Autodesk Inventor part; units mm, degrees
ref_plane "b1_XY" through (-12.7, 0, -12.7) normal (1, 0, 0) x (0, 0, -1)
ref_plane "b1_YZ" through (-12.7, 0, -12.7) normal (0, 0, -1) x (0, 1, 0)
ref_plane "b1_ZX" through (-12.7, 0, -12.7) normal (0, 1, 0) x (1, 0, 0)
sketch "Sketch_1" plane through (0, 0, 0) normal (0, 0, 1) x (1, 0, 0)
  arc A0 (-12.6998, -10.5664) -> (-10.5664, -12.6998) centre (-10.5918, -10.5918) ccw
  arc A1 (-9.5504, -12.7) -> (-10.5664, -12.6998) centre (-10.0584, -12.7) ccw
  line L0 (-9.5504, -12.7) -> (-6.3331, -12.7)
  arc A2 (-5.3171, -12.7) -> (-6.3331, -12.7) centre (-5.8251, -12.7) ccw
  line L1 (-5.3171, -12.7) -> (-4.3434, -12.7)
  arc A3 (-4.3434, -12.7) -> (-4.3434, -10.4902) centre (-4.3434, -11.5951) ccw
  line L2 (-4.3434, -10.4902) -> (-6.4748, -10.4902)
  arc A4 (-7.1932, -8.7558) -> (-6.4748, -10.4902) centre (-6.4748, -9.4742) ccw
  line L3 (-7.1932, -8.7558) -> (-3.8632, -5.4257)
  arc A5 (-1.6181, -4.4958) -> (-3.8632, -5.4257) centre (-1.6181, -7.6708) ccw
  line L4 (-1.6181, -4.4958) -> (1.6181, -4.4958)
  arc A6 (3.8632, -5.4257) -> (1.6181, -4.4958) centre (1.6181, -7.6708) ccw
  line L5 (3.8632, -5.4257) -> (7.1932, -8.7558)
  arc A7 (6.4748, -10.4902) -> (7.1932, -8.7558) centre (6.4748, -9.4742) ccw
  line L6 (6.4748, -10.4902) -> (4.3434, -10.4902)
  arc A8 (4.3434, -10.4902) -> (4.3434, -12.7) centre (4.3434, -11.5951) ccw
  line L7 (4.3434, -12.7) -> (5.3171, -12.7)
  arc A9 (6.3331, -12.7) -> (5.3171, -12.7) centre (5.8251, -12.7) ccw
  line L8 (6.3331, -12.7) -> (9.5504, -12.7)
  arc A10 (10.5664, -12.6998) -> (9.5504, -12.7) centre (10.0584, -12.7) ccw
  arc A11 (10.5664, -12.6998) -> (12.6998, -10.5664) centre (10.5918, -10.5918) ccw
  arc A12 (12.7, -9.5504) -> (12.6998, -10.5664) centre (12.7, -10.0584) ccw
  line L9 (12.7, -9.5504) -> (12.7, -6.3331)
  arc A13 (12.7, -5.3171) -> (12.7, -6.3331) centre (12.7, -5.8251) ccw
  line L10 (12.7, -5.3171) -> (12.7, -4.3434)
  arc A14 (12.7, -4.3434) -> (10.4902, -4.3434) centre (11.5951, -4.3434) ccw
  line L11 (10.4902, -4.3434) -> (10.4902, -6.4748)
  arc A15 (8.7558, -7.1932) -> (10.4902, -6.4748) centre (9.4742, -6.4748) ccw
  line L12 (8.7558, -7.1932) -> (5.4257, -3.8632)
  arc A16 (4.4958, -1.6181) -> (5.4257, -3.8632) centre (7.6708, -1.6181) ccw
  line L13 (4.4958, -1.6181) -> (4.4958, 1.6181)
  arc A17 (5.4257, 3.8632) -> (4.4958, 1.6181) centre (7.6708, 1.6181) ccw
  line L14 (5.4257, 3.8632) -> (8.7558, 7.1932)
  arc A18 (10.4902, 6.4748) -> (8.7558, 7.1932) centre (9.4742, 6.4748) ccw
  line L15 (10.4902, 6.4748) -> (10.4902, 4.3434)
  arc A19 (10.4902, 4.3434) -> (12.7, 4.3434) centre (11.5951, 4.3434) ccw
  line L16 (12.7, 4.3434) -> (12.7, 5.3171)
  arc A20 (12.7, 6.3331) -> (12.7, 5.3171) centre (12.7, 5.8251) ccw
  line L17 (12.7, 6.3331) -> (12.7, 9.5504)
  arc A21 (12.6998, 10.5664) -> (12.7, 9.5504) centre (12.7, 10.0584) ccw
  arc A22 (12.6998, 10.5664) -> (10.5664, 12.6998) centre (10.5918, 10.5918) ccw
  arc A23 (9.5504, 12.7) -> (10.5664, 12.6998) centre (10.0584, 12.7) ccw
  line L18 (9.5504, 12.7) -> (6.3331, 12.7)
  arc A24 (5.3171, 12.7) -> (6.3331, 12.7) centre (5.8251, 12.7) ccw
  line L19 (5.3171, 12.7) -> (4.3434, 12.7)
  arc A25 (4.3434, 12.7) -> (4.3434, 10.4902) centre (4.3434, 11.5951) ccw
  line L20 (4.3434, 10.4902) -> (6.4748, 10.4902)
  arc A26 (7.1932, 8.7558) -> (6.4748, 10.4902) centre (6.4748, 9.4742) ccw
  line L21 (7.1932, 8.7558) -> (3.8632, 5.4257)
  arc A27 (1.6181, 4.4958) -> (3.8632, 5.4257) centre (1.6181, 7.6708) ccw
  line L22 (1.6181, 4.4958) -> (-1.6181, 4.4958)
  arc A28 (-3.8632, 5.4257) -> (-1.6181, 4.4958) centre (-1.6181, 7.6708) ccw
  line L23 (-3.8632, 5.4257) -> (-7.1932, 8.7558)
  arc A29 (-6.4748, 10.4902) -> (-7.1932, 8.7558) centre (-6.4748, 9.4742) ccw
  line L24 (-6.4748, 10.4902) -> (-4.3434, 10.4902)
  arc A30 (-4.3434, 10.4902) -> (-4.3434, 12.7) centre (-4.3434, 11.5951) ccw
  line L25 (-4.3434, 12.7) -> (-5.3171, 12.7)
  arc A31 (-6.3331, 12.7) -> (-5.3171, 12.7) centre (-5.8251, 12.7) ccw
  line L26 (-6.3331, 12.7) -> (-9.5504, 12.7)
  arc A32 (-10.5664, 12.6998) -> (-9.5504, 12.7) centre (-10.0584, 12.7) ccw
  arc A33 (-10.5664, 12.6998) -> (-12.6998, 10.5664) centre (-10.5918, 10.5918) ccw
  arc A34 (-12.7, 9.5504) -> (-12.6998, 10.5664) centre (-12.7, 10.0584) ccw
  line L27 (-12.7, 9.5504) -> (-12.7, 6.3331)
  arc A35 (-12.7, 5.3171) -> (-12.7, 6.3331) centre (-12.7, 5.8251) ccw
  line L28 (-12.7, 5.3171) -> (-12.7, 4.3434)
  arc A36 (-12.7, 4.3434) -> (-10.4902, 4.3434) centre (-11.5951, 4.3434) ccw
  line L29 (-10.4902, 4.3434) -> (-10.4902, 6.4748)
  arc A37 (-8.7558, 7.1932) -> (-10.4902, 6.4748) centre (-9.4742, 6.4748) ccw
  line L30 (-8.7558, 7.1932) -> (-5.4257, 3.8632)
  arc A38 (-4.4958, 1.6181) -> (-5.4257, 3.8632) centre (-7.6708, 1.6181) ccw
  line L31 (-4.4958, 1.6181) -> (-4.4958, -1.6181)
  arc A39 (-5.4257, -3.8632) -> (-4.4958, -1.6181) centre (-7.6708, -1.6181) ccw
  line L32 (-5.4257, -3.8632) -> (-8.7558, -7.1932)
  arc A40 (-10.4902, -6.4748) -> (-8.7558, -7.1932) centre (-9.4742, -6.4748) ccw
  line L33 (-10.4902, -6.4748) -> (-10.4902, -4.3434)
  arc A41 (-10.4902, -4.3434) -> (-12.7, -4.3434) centre (-11.5951, -4.3434) ccw
  line L34 (-12.7, -4.3434) -> (-12.7, -5.3171)
  arc A42 (-12.7, -6.3331) -> (-12.7, -5.3171) centre (-12.7, -5.8251) ccw
  line L35 (-12.7, -6.3331) -> (-12.7, -9.5504)
  arc A43 (-12.6998, -10.5664) -> (-12.7, -9.5504) centre (-12.7, -10.0584) ccw
  circle A44 centre (0, 0) radius 2.6035
extrude "Extrusion1" add sketch "Sketch_1" against normal blind 248.6
ref_plane "b1_XY" through (-12.7, 0, -12.7) normal (1, 0, 0) x (0, 0, -1)
ref_plane "b1_YZ" through (-12.7, 0, -12.7) normal (0, 0, -1) x (0, 1, 0)
ref_plane "b1_ZX" through (-12.7, 0, -12.7) normal (0, 1, 0) x (1, 0, 0)
ref_plane "b2_XY" through (12.7, 0, -12.7) normal (1, 0, 0) x (0, 0, -1)
ref_plane "b2_YZ" through (12.7, 0, -12.7) normal (0, 0, -1) x (0, 1, 0)
ref_plane "b2_ZX" through (12.7, 0, -12.7) normal (0, 1, 0) x (1, 0, 0)
ref_plane "profile1010_XY" through (0, 0, -12.7) normal (0, 0, 1) x (1, 0, 0)
ref_plane "profile1010_YZ" through (0, 0, -12.7) normal (1, 0, 0) x (0, 1, 0)
ref_plane "profile1010_ZX" through (0, 0, -12.7) normal (0, 1, 0) x (0, 0, 1)
properties part number "1010_248_6mm"
Verification items for the finished model (mm, model axes). Give positions to 0.01 mm unless a question says otherwise; leave off trailing zeros. One line per question, with ' | ' between items.
1) Mould release check, pull along Y, two halves, no side actions. Record for faces 1 (the flat face through (0, 3, -248.6)), 2 (the cylindrical face through (2.483, 0.782, -122.56)): released by +Y, released by -Y, zero draft, split by the parting line, or undercut.
Result:
face 1: zero draft | face 2: undercut
2) Gauge pin test, flat ends, axial feed: pin 1 Ø1.6 at (y, z) = (0, -102) entering from +X; pin 2 Ø1.6 at (y, z) = (0.5, -132) entering from -X; pin 3 Ø2.5 at (x, z) = (-0.5, -113.5) entering from -Y. Record the tip position at first contact, or that the pin passes through.
Result:
pin 1: stops at x = 4.5 | pin 2: stops at x = -4.5 | pin 3: stops at y = -4.5
3) Thickness scan on line 1 along Y through (x, z) = (9.5, -17); line 2 along X through (y, z) = (-6.5, -28); line 3 along X through (y, z) = (6, -49). Record the ranges inside material, lowest first. Write a range as [from, to].
Result:
line 1: y = [-12.7, -7.49], [7.49, 12.7] | line 2: x = [-12.7, -10.49], [-8.06, -4.94], [4.94, 8.06], [10.49, 12.7] | line 3: x = [-12.22, -10.49], [-7.56, -4.44], [4.44, 7.56], [10.49, 12.22]
